```python
from build123d import *

# Parameters (mm, degrees)
SKETCH1_R           = 10
BOSS_EXTRUDE1_DEPTH = 506
SHELL1_T            = -2
BOSS_EXTRUDE2_START = -1
SKETCH2_R           = 15
SKETCH2_R_2         = 10
BOSS_EXTRUDE2_DEPTH = 4
LPATTERN1_COUNT     = 2
LPATTERN1_PITCH     = 499


with BuildPart() as part:
    # Sketch1 → Boss-Extrude1 (new body)
    with BuildSketch(Plane(origin=(0, 0, 0), x_dir=(1, 0, 0), z_dir=(0, 1, 0))):
        with Locations(Location((0, 0, 0), (0, 0, 270))):
            Circle(SKETCH1_R)
    extrude(amount=BOSS_EXTRUDE1_DEPTH)

    # Shell1
    shell1_openings = [part.faces().sort_by_distance(p)[0] for p in [
        (0, 506, 0),
        (0, 0, 0),
    ]]
    offset(amount=SHELL1_T, openings=shell1_openings, kind=Kind.INTERSECTION)

    # Sketch2 → Boss-Extrude2 (add)
    with BuildSketch(Plane(origin=(0, 506, 0), x_dir=(1, 0, 0), z_dir=(0, 1, 0)).offset(BOSS_EXTRUDE2_START)):
        with Locations(Location((0, 0, 0), (0, 0, 270))):
            Circle(SKETCH2_R)
        with Locations(Location((0, 0, 0), (0, 0, 270))):
            Circle(SKETCH2_R_2, mode=Mode.SUBTRACT)
    boss_extrude2 = extrude(amount=BOSS_EXTRUDE2_DEPTH)

    # LPattern1: Boss-Extrude2 ×2
    with Locations(*[(0, -i * LPATTERN1_PITCH, 0) for i in range(1, LPATTERN1_COUNT)]):
        add(boss_extrude2)


solid = part.part
```
For this review, take the finished solid that the model builds, in its own axes (mm). A direction names the side the tool comes from. Coordinates: 2 decimals unless noted, no trailing zeros. Write each loop counter-clockwise with the first axis right and the second up, starting at its lowest first coordinate (ties: lowest second). Pieces come first, ordered by that corner, then holes. Notation, with made-up numbers: (80.25, 65.25) - (135.25, 65.25) arc R27 ccw to (135.25, 95.25) - close; hole circle Ø7 at (4.5, 49). An arc over 180 degrees is marked (long way). Put each result on its own line as item: value.
1. Wall thickness on probe 1 along X at (y, z) = (334, 0); probe 2 along Y at (x, z) = (9.25, -8); probe 3 along X at (y, z) = (485, 1.25): over which ranges is each line inside the solid? List them lowest first.
Values found:
probe 1: -10 to -8, 8 to 10
probe 2: 6 to 10, 505 to 509
probe 3: -9.92 to -7.9, 7.9 to 9.92
2. For pin 1 (15 mm diameter, centred on x = -3, z = 5, fed in from -Y); pin 2 (6 mm diameter, centred on y = 194, z = -7, fed in from -X); pin 3 (14.5 mm diameter, centred on x = 0, z = 0, fed in from -Y); pin 4 (8 mm diameter, centred on y = 163.5, z = -9.5, fed in from +X), all flat-tipped, find the tip position at first contact; note any pin that passes through.
Values found:
pin 1: y = 0
pin 2: x = -9.17
pin 3: through
pin 4: x = 8.35
3. Add section B-B, the plane x = 0. Give the boundary of the cut face in (y, z).
Values found:
outline: (0, -10) - (6, -10) - (6, -15) - (10, -15) - (10, -10) - (505, -10) - (505, -15) - (509, -15) - (509, -10) - (506, -10) - (506, -8) - (0, -8) - close; (0, 8) - (506, 8) - (506, 10) - (509, 10) - (509, 15) - (505, 15) - (505, 10) - (10, 10) - (10, 15) - (6, 15) - (6, 10) - (0, 10) - close
4. Add section A-A, the plane z = 0. Give the boundary of the cut face in (x, y), then the cut area to 3 significant figures.
Values found:
outline: (-15, 6) - (-10, 6) - (-10, 0) - (-8, 0) - (-8, 506) - (-10, 506) - (-10, 509) - (-15, 509) - (-15, 505) - (-10, 505) - (-10, 10) - (-15, 10) - close; (8, 0) - (10, 0) - (10, 6) - (15, 6) - (15, 10) - (10, 10) - (10, 505) - (15, 505) - (15, 509) - (10, 509) - (10, 506) - (8, 506) - close
area: 2,100 mm²
5. Machinability: for faces 1 (the cylindrical face through (0.66, 7.972, -14.985)), 2 (the flat face through (8.2, 0, 0)), 3 (the flat face through (-10, 6, 3)), 4 (the cylindrical face through (-9.76, 507.48, -2.17)), 5 (the cylindrical face through (-9.76, 254.04, -2.17)), which of the approach directions +Z, -Z, +X, -X, +Y, -Y give a long, thin tool a straight path to every point of the face, cutting with its end or side? Answer none if there is none.
Values found:
face 1: +Y, -Y
face 2: +Z, -Z, +X, -X, -Y
face 3: -Y
face 4: +Y
face 5: none
6. Add section C-C, the plane y = 58.5. Give the boundary of the cut face in (x, z), then the cut area to 3 significant figures.
Values found:
outline: circle Ø20 at (0, 0); hole circle Ø16 at (0, 0)
area: 113 mm²
7. Mouldability with a two-part tool opening along Z and no side actions: class faces 6 (the cylindrical face through (0.66, 506.972, -14.985)), 7 (the flat face through (8.2, 506, 0)), 8 (the flat face through (-10, 509, 3)) as released by +Z, released by -Z, zero draft, split by the parting line, or undercut.
Values found:
face 6: split by the parting line
face 7: undercut
face 8: zero draft
